Autodesk Inventor part; units mm, degrees
ref_plane "YZ Plane" through (0, 0, 0) normal (1, 0, 0) x (0, 1, 0)
ref_plane "XZ Plane" through (0, 0, 0) normal (0, 1, 0) x (-1, 0, 0)
ref_plane "XY Plane" through (0, 0, 0) normal (0, 0, 1) x (1, 0, 0)
sketch "Sketch1" plane through (0, 0, 0) normal (0, 0, 1) x (1, 0, 0)
  circle A0 centre (0, 0) radius 35
  dimension "d0" = 70
extrude "Extrusion1" add sketch "Sketch1" along normal blind 21
sketch "Sketch2" plane through (0, 0, 21) normal (0, 0, 1) x (1, 0, 0)
  circle A0 centre (0, 0) radius 6.75
  dimension "d3" = 13.5
extrude "Extrusion2" add sketch "Sketch2" along normal blind 5
sketch "Sketch3" plane through (0, 0, 26) normal (0, 0, 1) x (1, 0, 0)
  line L0 (-11.5, -10) -> (11.5, -10)
  line L1 (11.5, -10) -> (11.5, 32)
  line L2 (11.5, 32) -> (-11.5, 32)
  line L3 (-11.5, 32) -> (-11.5, -10)
  point P0 (0, 0)
  point P1 (0, -10)
  dimension "d6" = 42
  dimension "d7" = 23
  dimension "d8" = 10
extrude "Extrusion3" add sketch "Sketch3" along normal blind 45
sketch "Sketch4" plane through (-11.5, -10, 26) normal (-1, 0, 0) x (0, 0, 1)
  line L0 (0, 0) -> (0, 42)
  line L1 (0, 42) -> (45, 42)
  line L2 (0, 0) -> (15, 0)
  line L3 (15, 0) -> (15, 42)
  line L4 (15, 42) -> (0, 42)
  line L5 (0, 42) -> (0, 0)
  point P0 (-26, 10)
  dimension "d11" = 15
extrude "Extrusion4" add sketch "Sketch4" along normal blind 1.5
sketch "Sketch5" plane through (-11.5, 32, 71) normal (0, 1, 0) x (1, 0, 0)
  line L0 (-1.5, 45) -> (-1.5, 30)
  line L1 (-1.5, 30) -> (23, 30)
  line L2 (23, 30) -> (23, 45)
  line L3 (23, 45) -> (-1.5, 45)
  line L4 (-1.5, 45) -> (-1.5, 30)
  point P0 (11.5, 71)
extrude "Extrusion5" add sketch "Sketch5" along normal blind 1.5
sketch "Sketch6" plane through (-11.5, -10, 71) normal (0, -1, 0) x (1, 0, 0)
  line L0 (23, -30) -> (0, -30)
  line L1 (-1.5, -45) -> (23, -45)
  line L2 (23, -45) -> (23, -30)
  line L3 (23, -30) -> (-1.5, -30)
  line L4 (-1.5, -30) -> (-1.5, -45)
  point P0 (11.5, -71)
extrude "Extrusion6" add sketch "Sketch6" along normal blind 1.5
sketch "Sketch7" plane through (-11.5, -11.5, 71) normal (0, -1, 0) x (1, 0, 0)
  line L0 (23, -45) -> (-1.5, -45)
  line L1 (-1.5, -30) -> (23, -30)
  line L2 (23, -45) -> (21.5, -45)
  line L3 (21.5, -45) -> (21.5, -30)
  line L4 (21.5, -30) -> (23, -30)
  line L5 (23, -30) -> (23, -45)
  point P0 (11.5, -71)
  dimension "d18" = 1.5
extrude "Extrusion7" add sketch "Sketch7" along normal blind 16
sketch "Sketch8" plane through (-11.5, 33.5, 71) normal (0, 1, 0) x (1, 0, 0)
  line L0 (-1.5, 45) -> (21.5, 45)
  line L1 (23, 30) -> (21.5, 30)
  line L2 (21.5, 30) -> (21.5, 45)
  line L3 (21.5, 45) -> (23, 45)
  line L4 (23, 45) -> (23, 30)
  point P0 (11.5, 71)
  dimension "d21" = 1.5
extrude "Extrusion8" add sketch "Sketch8" along normal blind 16
sketch "Sketch9" plane through (0, 0, 0) normal (0, 0, -1) x (-1, 0, 0)
  circle A0 centre (0, 0) radius 1.25
  dimension "d24" = 2.5
extrude "Extrusion9" cut sketch "Sketch9" against normal blind 50
properties part number "Rueda Derecha"
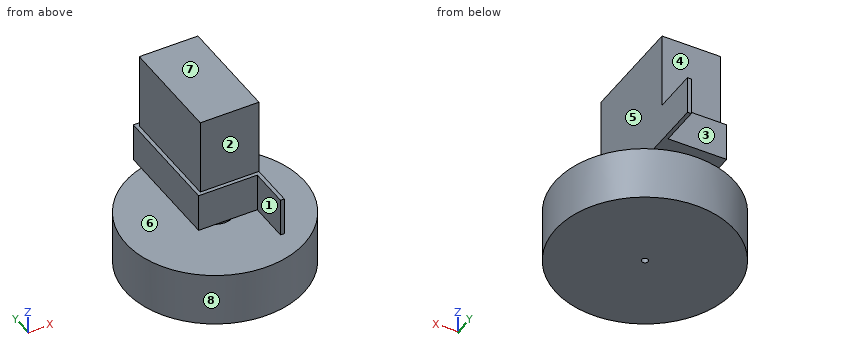
Part model, mm, in its own coordinate system. Face numbers are marked on the shaded views. A direction names the side the tool comes from. Give positions to 0.01 mm unless a question says otherwise; leave off trailing zeros. Order: outer loops, then holes, each group sorted by start corner. A loop starts at its lowest first (then second) coordinate and runs counter-clockwise, first axis right, second up. Notation, with made-up numbers: M -1.75,9 L 51.25,9 A20 ccw 51.25,13 Z; hole C 24.25,23.25 d1. An arc over 180 degrees is marked long. Use a Markdown table: item, result. Add a question column.
(1) 3-axis set-ups, long thin cutter, end or side, ignore diameter. For the marked faces 1, 2, 3, 4 and 5: which of +Z, -Z, +X, -X, +Y, -Y reach the whole face in a straight line?
(2) Saw through at A-A, the plane x = 0. Give the cut face in (y, z), and give its area (3 significant figures).
(3) Mould opens along Z. For the marked faces 6, 7 and 8 say: +Z half, -Z half, draft (parallel to the pull), parting line (faces both ways), or undercut.
(4) Saw through at C-C, the plane z = 39. Give the cut face in (x, y), and give its area (3 significant figures).
(5) Probe line 1 along Y through (x, z) = (0, 24); line 2 along Y through (x, z) = (0, 35); line 3 along Z through (x, y) = (9, -4). List the from-to ranges inside material, lowest first. Write a range as [from, to].
(6) Saw through at B-B, the plane y = 0. Give the cut face in (x, z).
(7) Drop flat-ended pins along their axis: P1, Ø10, axis at y = 35, z = 28.5, coming from the -X side; P2, Ø2, axis at y = 3, z = 41, coming from the +X side; P3, Ø3, axis at x = 8.5, z = 57, coming from the -Y side. Give the stop position or say it passes through.
(8) Saw through at D-D, the plane x = 8.5. Give the cut face in (y, z), and give its area (3 significant figures).
Answer key:
| question | item | result |
|---|---|---|
| 1 | face 1 | +Z, -X, -Y |
| 1 | face 2 | +Z, +X, -X, -Y |
| 1 | face 3 | +Z, -X, +Y |
| 1 | face 4 | +Z, +X, -X, +Y |
| 1 | face 5 | +Z, +X, +Y, -Y |
| 2 | outline | M -35,0 L -1.25,0 L -1.25,50 L 1.25,50 L 1.25,0 L 35,0 L 35,21 L 6.75,21 L 6.75,26 L 33.5,26 L 33.5,41 L 32,41 L 32,71 L -10,71 L -10,41 L -11.5,41 L -11.5,26 L -6.75,26 L -6.75,21 L -35,21 Z |
| 2 | area | 3,350 mm^2 |
| 3 | face 6 | undercut |
| 3 | face 7 | +Z half |
| 3 | face 8 | draft |
| 4 | outline | M -13,-11.5 L 10,-11.5 L 10,-27.5 L 11.5,-27.5 L 11.5,49.5 L 10,49.5 L 10,33.5 L -13,33.5 Z; hole C 0,0 d2.5 |
| 4 | area | 1,150 mm^2 |
| 5 | line 1 | [-6.75, -1.25], [1.25, 6.75] |
| 5 | line 2 | [-11.5, -1.25], [1.25, 33.5] |
| 5 | line 3 | [0, 21], [26, 71] |
| 6 | outline | M -35,0 L -1.25,0 L -1.25,50 L 1.25,50 L 1.25,0 L 35,0 L 35,21 L 6.75,21 L 6.75,26 L 11.5,26 L 11.5,71 L -11.5,71 L -11.5,41 L -13,41 L -13,26 L -6.75,26 L -6.75,21 L -35,21 Z |
| 7 | P1 | x = -13 |
| 7 | P2 | x = 11.5 |
| 7 | P3 | y = -10 |
| 8 | outline | M -33.95,0 L 33.95,0 L 33.95,21 L -33.95,21 Z; M -11.5,26 L 33.5,26 L 33.5,41 L 32,41 L 32,71 L -10,71 L -10,41 L -11.5,41 Z |
| 8 | area | 3,360 mm^2 |
